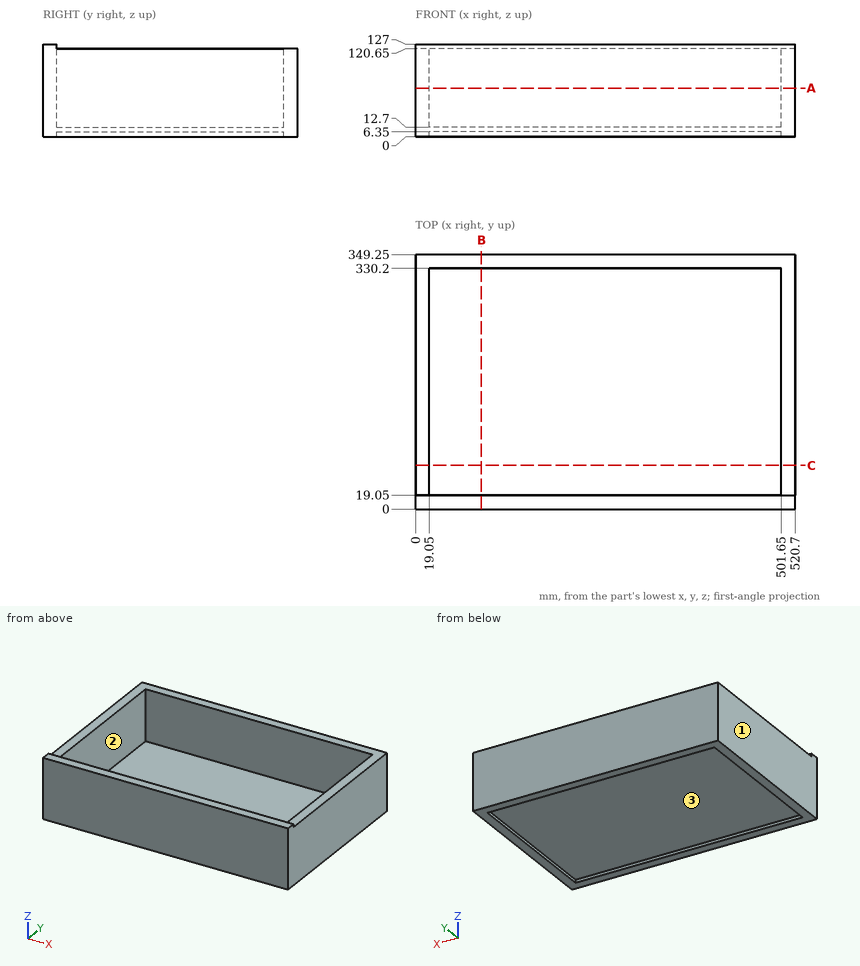
Here's the drawing with two shaded views (mm, measured from the low corner). I have some questions. A direction names the side the tool comes from. Round coordinates to 2 decimals unless told otherwise and drop trailing zeros. Loops run counter-clockwise (first coordinate to the right, second up) from the corner with the lowest first, then second, coordinate; pieces in that order, holes last. Notation, with made-up numbers: (5, -38.5) - (39, -38.5) arc R21 ccw to (39, -18.5) - close; hole circle Ø2 at (5.5, 89). An arc over 180 degrees is marked (long way). Use CSV: the item, a comma, the result in double quotes. Start each with the question number.
1) If we section it at C-C on y = 60: Write out the boundary of the cut face in (x, z), plus the area to 3 significant figures.
2) For the marked faces 1, 2 and 3, which set-ups out of +Z, -Z, +X, -X, +Y, -Y let a thin tool reach every point of the face, with its end or its side?
3) Please list where these lines run through material, in increasing order: probe 1 along Y at (x, z) = (382.5, 53); probe 2 along X at (y, z) = (212.5, 63); probe 3 along Z at (x, y) = (227, 156.5). Write a range as [from, to].
4) If we section it at B-B on x = 90.5: Write out the boundary of the cut face in (y, z), plus the area to 3 significant figures.
5) If we section it at A-A on z = 66.5: Write out the boundary of the cut face in (x, y), plus the area to 3 significant figures.
6) For pin 1 Ø5 at (x, y) = (156, 135.5) entering from +Z; pin 2 Ø6 at (x, y) = (66, 222) entering from -Z, each with a flat end and sliding along its axis, tell me the tip position at first contact or that it passes through.
Geometry results:
1,outline,"(0, 0) - (19.05, 0) - (19.05, 6.35) - (501.65, 6.35) - (501.65, 0) - (520.7, 0) - (520.7, 120.65) - (501.65, 120.65) - (501.65, 12.7) - (19.05, 12.7) - (19.05, 120.65) - (0, 120.65) - close"
1,area,"7,660 mm2"
2,face 1,"+Z, -Z, -X, +Y, -Y"
2,face 2,"+Z"
2,face 3,"-Z"
3,probe 1,"y = [0, 19.05], [330.2, 349.25]"
3,probe 2,"x = [0, 19.05], [501.65, 520.7]"
3,probe 3,"z = [6.35, 12.7]"
4,outline,"(0, 0) - (19.05, 0) - (19.05, 6.35) - (330.2, 6.35) - (330.2, 0) - (349.25, 0) - (349.25, 120.65) - (330.2, 120.65) - (330.2, 12.7) - (19.05, 12.7) - (19.05, 127) - (0, 127) - close"
4,area,"6,690 mm2"
5,outline,"(0, 0) - (520.7, 0) - (520.7, 349.25) - (0, 349.25) - close; hole (19.05, 19.05) - (501.65, 19.05) - (501.65, 330.2) - (19.05, 330.2) - close"
5,area,"31,700 mm2"
6,pin 1,"stops at z = 12.7"
6,pin 2,"stops at z = 6.35"
